Part model, mm, in its own coordinate system. A direction names the side the tool comes from. Round coordinates to 2 decimals unless told otherwise and drop trailing zeros. Loops run counter-clockwise (first coordinate to the right, second up) from the corner with the lowest first, then second, coordinate; pieces in that order, holes last. Notation, with made-up numbers: (9, 13.25) -> (40, 13.25) arc R23 ccw to (40, 34.25) -> close; hole circle Ø2 at (-11, 5.25). An arc over 180 degrees is marked (long way). Use a Markdown table: item, result. Add a question column.
Item 1: Two-plate mould, pull along Y, no slides. Class faces 1 (the face through (0, -20.5, 21)), 2 (the face through (7.72, 8.25, 0.74)), 3 (the face through (0, -12, 1.5)): pulls with the +Y half, pulls with the -Y half, needs draft (parallel to the pull), parting line crosses it, or undercut.
Item 2: Cut at B-B, the plane z = 35. List the corners of the cut face in (x, y), plus the area to 3 significant figures.
Item 3: Cut at A-A, the plane x = 0. List the corners of the cut face in (y, z), plus the area to 3 significant figures.
Item 4: Which spindle directions (+Z, -Z, +X, -X, +Y, -Y) get a long thin tool onto all of the face, cutting with end or side? Do faces 4 (the face through (0, -20, 40)), 5 (the face through (0, -19, 21)). Say none if no direction does.
Item 5: Probe line 1 (X direction, y = -19.55, z = 15); line 2 (Z direction, x = 15.5, y = -19.45); line 3 (Z direction, x = 15.5, y = -19.7). List the from-to ranges inside material, lowest first. Write a range as [from, to].
Item 6: Cut at D-D, the plane y = -15.5. List the corners of the cut face in (x, z), plus the area to 3 significant figures.
Item 7: Cut at C-C, the plane x = 15.5. List the corners of the cut face in (y, z).
Item 8: Flat gauge pins, fed straight in: pin 1 (4 mm diameter, centred on x = -15.5, z = 15, fed in from -Y); pin 2 (2 mm diameter, centred on x = 15.5, z = 35, fed in from -Y); pin 3 (4 mm diameter, centred on x = 5, z = 6.5, fed in from +Y); pin 4 (8 mm diameter, centred on x = -8.5, y = 11.5, fed in from +Z). Where does each tip first touch, or does it go through?
Autodesk Inventor part; units mm, degrees
ref_plane "YZ Plane" through (0, 0, 0) normal (1, 0, 0) x (0, 1, 0)
ref_plane "XZ Plane" through (0, 0, 0) normal (0, 1, 0) x (-1, 0, 0)
ref_plane "XY Plane" through (0, 0, 0) normal (0, 0, 1) x (1, 0, 0)
sketch "Sketch1" plane through (0, 0, 0) normal (0, 0, 1) x (1, 0, 0)
  line L0 (20, 0) -> (20, -20.5)
  line L1 (20, -20.5) -> (-20, -20.5)
  line L2 (-20, -20.5) -> (-20, 0)
  arc A0 (20, 0) -> (-20, 0) centre (0, 0) ccw
  circle A1 centre (0, 0) radius 10.5
  dimension "d1" = 40
  dimension "d4" = 20
  dimension "d5" = 20.5
  dimension "d7" = 21
  dimension "d8" = 20
  dimension "MotorCenterOffset" = 20.5
extrude "Plate1" add sketch "Sketch1" along normal blind 1.5
sketch "Sketch3" plane through (20, -19, 0) normal (0, -1, 0) x (1, 0, 0)
  line L0 (-40, 0) -> (0, 0)
  line L1 (0, 0) -> (0, 40)
  line L2 (0, 40) -> (-40, 40)
  line L3 (-40, 40) -> (-40, 0)
edge flange "Flange1" height 40 angle 90 thickness 1.5 bend radius 0.5 thickness toward (0, -1, 0) relief tear relief width 1.5 relief depth 0.75 edges at (0, -20.5, 1.5) wall of the first edge with corners at (-20, -19, 0) (20, -19, 0) (20, -19, 40) (-20, -19, 40)
bend "Bend1"
corner "Corner1"
fillet "Corner Round1" radius 2 1 edges at (-20, -19.75, 40)
fillet "Corner Round1" radius 2 1 edges at (20, -19.75, 40)
sketch "Sketch4" plane through (-20, -19, 2) normal (0, 1, 0) x (1, 0, 0)
  line L0 (2, -38) -> (38, -38)
  line L1 (0, -36) -> (0, 0)
  line L2 (0, -33) -> (4.5, -33)
  line L3 (4.5, -33) -> (4.5, -38)
  point P0 (20, 2)
  dimension "d43" = 4.5
  dimension "d44" = 5
hole "Hole2" at (-15.5, -19, 35) direction (0, -1, 0) diameter 3.5 end through all
pattern_linear "Rectangular Pattern2" count 4 spacing 10 along (0, 0, -1) count 2 spacing 31 along (1, 0, 0) of "Hole2"
sketch "Sketch5" plane through (0, 0, 1.5) normal (0, 0, 1) x (1, 0, 0)
  line L0 (-20, -18.5) -> (-20, 0)
  circle A0 centre (0, 0) radius 10.5
  line L1 (0, 0) -> (9.1924, 9.1924)
  circle A1 centre (0, 0) radius 13
  line L2 (0, 0) -> (13, 0)
  circle A2 centre (9.1924, 9.1924) radius 1.75
  dimension "d59" = 26
  dimension "d60" = 45
  dimension "d61" = 3.5
hole "Hole3" at (9.1924, 9.1924, 1.5) direction (0, 0, -1) diameter 3.5 end through all
pattern_circular "Circular Pattern1" count 4 over 360 about axis through (0, 0, 0) along (0, 0, 1) of "Hole3"
equation "\"d50\" = Thickness"
equation "\"d12\" = BendReliefWidth"
equation "\"d13\" = BendReliefDepth"
equation "\"d14\" = MinimumRemnant"
equation "\"d15\" = BendRadius"
equation "\"d19\" = CornerReliefSize"
equation "\"d20\" = GapSize"
equation "\"d21\" = JacobiRadiusSize"
equation "\"BendRadius\" = Thickness"
equation "\"BendReliefWidth\" = Thickness"
equation "\"BendReliefDepth\" = 0.5 * Thickness"
equation "\"CornerReliefSize\" = 4 * Thickness"
equation "\"MinimumRemnant\" = 2 * Thickness"
equation "\"TransitionRadius\" = BendRadius"
equation "\"JacobiRadiusSize\" = BendRadius"
equation "\"GapSize\" = Thickness"
equation "\"d10\" = BendRadius"
properties part number "HD-BK-IG" material "Galvanized Steel"
A:
| question | item | result |
|---|---|---|
| 1 | face 1 | pulls with the -Y half |
| 1 | face 2 | undercut |
| 1 | face 3 | needs draft |
| 2 | outline | (-20, -20.5) -> (-17.25, -20.5) -> (-17.25, -19) -> (-20, -19) -> close; (-13.75, -20.5) -> (13.75, -20.5) -> (13.75, -19) -> (-13.75, -19) -> close; (17.25, -20.5) -> (20, -20.5) -> (20, -19) -> (17.25, -19) -> close |
| 2 | area | 49.5 mm^2 |
| 3 | outline | (-20.5, 2) arc R2 ccw to (-18.5, 0) -> (-10.5, 0) -> (-10.5, 1.5) -> (-18.5, 1.5) arc R0.5 cw to (-19, 2) -> (-19, 40) -> (-20.5, 40) -> close; (10.5, 0) -> (20, 0) -> (20, 1.5) -> (10.5, 1.5) -> close |
| 3 | area | 86.2 mm^2 |
| 4 | face 4 | +Z, +X, -X, +Y, -Y |
| 4 | face 5 | +Z, +X, -X, +Y |
| 5 | line 1 | x = [-20, -17.25], [-13.75, 13.75], [17.25, 20] |
| 5 | line 2 | z = [0.24, 3.25], [6.75, 13.25], [16.75, 23.25], [26.75, 33.25], [36.75, 40] |
| 5 | line 3 | z = [0.4, 3.25], [6.75, 13.25], [16.75, 23.25], [26.75, 33.25], [36.75, 40] |
| 6 | outline | (-20, 0) -> (20, 0) -> (20, 1.5) -> (-20, 1.5) -> close |
| 6 | area | 60.0 mm^2 |
| 7 | outline | (-20.5, 2) arc R2 ccw to (-18.5, 0) -> (12.64, 0) -> (12.64, 1.5) -> (-18.5, 1.5) arc R0.5 cw to (-19, 2) -> (-19, 3.25) -> (-20.5, 3.25) -> close; (-20.5, 6.75) -> (-19, 6.75) -> (-19, 13.25) -> (-20.5, 13.25) -> close; (-20.5, 16.75) -> (-19, 16.75) -> (-19, 23.25) -> (-20.5, 23.25) -> close; (-20.5, 26.75) -> (-19, 26.75) -> (-19, 33.25) -> (-20.5, 33.25) -> close; (-20.5, 36.75) -> (-19, 36.75) -> (-19, 40) -> (-20.5, 40) -> close |
| 8 | pin 1 | stops at y = -20.5 |
| 8 | pin 2 | passes through |
| 8 | pin 3 | stops at y = -19 |
| 8 | pin 4 | stops at z = 1.5 |
